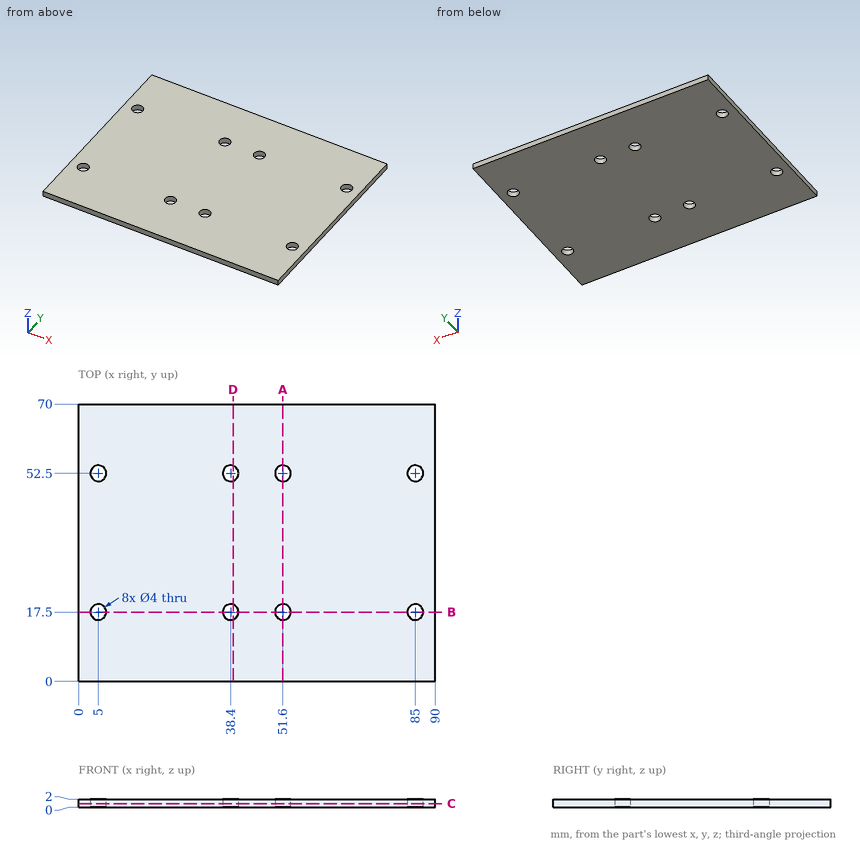
Could you check a few things on this drawing? It's one solid part, dimensions in mm from its lowest x, y, z. Coordinates: 2 decimals unless noted, no trailing zeros. Order: outer loops, then holes, each group sorted by start corner. A loop starts at its lowest first (then second) coordinate and runs counter-clockwise, first axis right, second up. Notation, with made-up numbers: (-28.75, -25.5) -> (-14.75, -25.5) arc R23 cw to (-14.75, -11.5) -> close; hole circle Ø10 at (27.25, 49.25). An arc over 180 degrees is marked (long way). One line per item, written item: value. Start each with the question number.
1) Imagine slicing it at C-C on z = 0.95. Count the separate pieces of the cut face and the enclosed holes in it, plus the area to 3 significant figures.
2) Imagine slicing it at D-D on x = 39. List the corners of the cut face in (y, z) for me, plus the area to 3 significant figures.
3) Imagine slicing it at A-A on x = 51.6. List the corners of the cut face in (y, z) for me, plus the area to 3 significant figures.
4) If I drill on L1, parallel to Y at x = 85, z = 0.6, over which ranges is the centre line in solid material (lowest first)? Write a range as [from, to].
5) Imagine slicing it at B-B on y = 17.5. List the corners of the cut face in (x, z) for me.
Answer list:
1. separate pieces: 1
1. enclosed holes: 8
1. area: 6,200 mm2
2. outline: (0, 0) -> (15.59, 0) -> (15.59, 2) -> (0, 2) -> close; (19.41, 0) -> (50.59, 0) -> (50.59, 2) -> (19.41, 2) -> close; (54.41, 0) -> (70, 0) -> (70, 2) -> (54.41, 2) -> close
2. area: 125 mm2
3. outline: (0, 0) -> (15.5, 0) -> (15.5, 2) -> (0, 2) -> close; (19.5, 0) -> (50.5, 0) -> (50.5, 2) -> (19.5, 2) -> close; (54.5, 0) -> (70, 0) -> (70, 2) -> (54.5, 2) -> close
3. area: 124 mm2
4. L1: y = [0, 15.5], [19.5, 50.5], [54.5, 70]
5. outline: (0, 0) -> (3, 0) -> (3, 2) -> (0, 2) -> close; (7, 0) -> (36.4, 0) -> (36.4, 2) -> (7, 2) -> close; (40.4, 0) -> (49.6, 0) -> (49.6, 2) -> (40.4, 2) -> close; (53.6, 0) -> (83, 0) -> (83, 2) -> (53.6, 2) -> close; (87, 0) -> (90, 0) -> (90, 2) -> (87, 2) -> close
